```python
from build123d import *

# Parameters (mm, degrees)
SZKIC1_R                    = 4.05
DODANIE_WYCI_GNI_CIE3_DEPTH = 1
SZKIC5_W                    = 6
SZKIC5_H                    = 1
DODANIE_WYCI_GNI_CIE5_DEPTH = 6
ZAOKR_GLENIE3_R             = 0.5


with BuildPart() as part:
    # Szkic1 → Dodanie-wyciągnięcie3 (new body)
    with BuildSketch(Plane.XY):
        with BuildLine():
            Line((3, 11.644169223), (-3, 11.644169223))
            Line((-3, 11.644169223), (-3, 9.644169223))
            ThreePointArc((-3, 9.644169223), (0, -10.1), (3, 9.644169223))
            Line((3, 9.644169223), (3, 11.644169223))
        make_face()
        Circle(SZKIC1_R, mode=Mode.SUBTRACT)
    extrude(amount=DODANIE_WYCI_GNI_CIE3_DEPTH)

    # Szkic5 → Dodanie-wyciągnięcie5 (add)
    with BuildSketch(Plane(origin=(0, 0, 0), x_dir=(-1, 0, 0), z_dir=(0, 0, -1))):
        with Locations((0, 11.144169223)):
            Rectangle(SZKIC5_W, SZKIC5_H)
    extrude(amount=DODANIE_WYCI_GNI_CIE5_DEPTH)

    # Zaokrąglenie3
    zaokr_glenie3_edges = [part.edges().sort_by_distance(p)[0] for p in [
        (-3, 9.644169223, 0.5),
        (3, 9.644169223, 0.5),
        (0, 11.644169223, -6),
        (0, 10.644169223, -6),
        (0, 10.644169223, 0),
        (0, 11.644169223, 1),
    ]]
    fillet(zaokr_glenie3_edges, radius=ZAOKR_GLENIE3_R - 0.0001)  # a hair under: the kernel refuses the full size


solid = part.part
```
Could you check a few things on this model? Use its own coordinates, in mm. A direction names the side the tool comes from. Give positions to 0.01 mm unless a question says otherwise; leave off trailing zeros. Loops run counter-clockwise (first coordinate to the right, second up) from the corner with the lowest first, then second, coordinate; pieces in that order, holes last. Notation, with made-up numbers: (45, 9.5) -> (53, 9.5) arc R22 ccw to (53, 31.5) -> close; hole circle Ø8 at (11.5, 61). An arc over 180 degrees is marked (long way). Put each result on its own line as item: value.
(1) Thinking about a two-plate mould opening in X: for faces 4 (the face through (3, 11, -2)), 5 (the face through (0, 11.644, -2)), 6 (the face through (-0.878, -3.954, 0.493)), which applies, pulls with the +X half, pulls with the -X half, needs draft (parallel to the pull), parting line crosses it, or undercut?
Computed:
face 4: pulls with the +X half
face 5: needs draft
face 6: undercut
(2) Please list where these lines run through material, in increasing order: probe 1 along Y at (x, z) = (0, 0.5); probe 2 along Y at (x, z) = (-0.5, -5.5); probe 3 along Z at (x, y) = (7.5, -3.5). Write a range as [from, to].
Computed:
probe 1: [-10.1, -4.05], [4.05, 11.64]
probe 2: [10.64, 11.64]
probe 3: [0, 1]
(3) Imagine slicing it at D-D on y = -3.5. Write out the boundary of the cut face in (x, z), plus the area to 3 significant figures.
Computed:
outline: (-9.47, 0) -> (-2.04, 0) -> (-2.04, 1) -> (-9.47, 1) -> close; (2.04, 0) -> (9.47, 0) -> (9.47, 1) -> (2.04, 1) -> close
area: 14.9 mm^2
(4) Imagine slicing it at C-C on z = -0.75. Write out the boundary of the cut face in (x, y), plus the area to 3 significant figures.
Computed:
outline: (-3, 10.64) -> (3, 10.64) -> (3, 11.64) -> (-3, 11.64) -> close
area: 6.00 mm^2
(5) I'm going to push flat-ended pins straight in: pin 1 Ø2 at (x, y) = (-2, 8.5) entering from -Z; pin 2 Ø0.5 at (y, z) = (10.5, -3) entering from -X; pin 3 Ø10 at (x, y) = (-4, 6) entering from -Z. Where does each tip first touch, or does it pass through?
Computed:
pin 1: z = 0
pin 2: x = -3
pin 3: z = -5.94
(6) Imagine slicing it at A-A on y = 0. Write out the boundary of the cut face in (x, z), plus the area to 3 significant figures.
Computed:
outline: (-10.1, 0) -> (-4.05, 0) -> (-4.05, 1) -> (-10.1, 1) -> close; (4.05, 0) -> (10.1, 0) -> (10.1, 1) -> (4.05, 1) -> close
area: 12.1 mm^2
(7) For faces 1 (the face through (0, 10.644, -3)), 2 (the face through (-3, 11, -2)), 3 (the face through (-2, -4, 1)), which set-ups out of +Z, -Z, +X, -X, +Y, -Y let a thin tool reach every point of the face, with its end or its side?
Computed:
face 1: -Z, +X, -X, -Y
face 2: +Z, -Z, -X, +Y
face 3: +Z, +X, -X, +Y, -Y
